```python
from build123d import *

# Parameters (mm, degrees)
BOSS_EXTRUDE1_DEPTH        = 3
BOSS_EXTRUDE1_DEPTH_BACK   = 3
SKETCH2_R                  = 4.5
BOSS_EXTRUDE2_DEPTH        = 8.5
BOSS_EXTRUDE2_DEPTH_BACK   = 8.5
SKETCH2_4_R                = 4.5
BOSS_EXTRUDE3_DEPTH        = 8.5
BOSS_EXTRUDE3_DEPTH_BACK   = 8.5
M3_TAPPED_HOLE1_REACH      = 52.91
M3_TAPPED_HOLE1_BORE_R     = 1.25
M3_TAPPED_HOLE2_REACH      = 52.91
M3_TAPPED_HOLE2_BORE_R     = 1.25
M4_TAPPED_HOLE1_AT_2_COUNT = 2
M4_TAPPED_HOLE1_AT_2_PITCH = 12
M5_TAPPED_HOLE2_AT_2_COUNT = 2
M5_TAPPED_HOLE2_AT_2_PITCH = 12


with BuildPart() as part:
    # Sketch2 → Boss-Extrude1 (new, two sides: drawn at the far end of the back side and taken through both)
    with BuildSketch(Plane(origin=(0, 0, 0), x_dir=(0, 0, -1), z_dir=(1, 0, 0)).offset(-BOSS_EXTRUDE1_DEPTH_BACK)):
        with BuildLine():
            Line((-6, -4.733334115), (20.564415122, -14.401990511))
            ThreePointArc((20.564415122, -14.401990511), (27.686806127, -12.56566856), (28.53576338, -5.259520223))
            ThreePointArc((28.53576338, -5.259520223), (28.211096751, -4.433651902), (28.076506478, -3.556524566))
            ThreePointArc((28.076506478, -3.556524566), (27.692579293, -2.458130667), (26.76223606, -1.759324035))
            Line((26.76223606, -1.759324035), (23.943158198, -0.733263605))
            ThreePointArc((23.943158198, -0.733263605), (23.371504837, -0.615809048), (22.790282203, -0.668376983))
            ThreePointArc((22.790282203, -0.668376983), (21.627836935, -0.773512852), (20.484530213, -0.538603739))
            Line((20.484530213, -0.538603739), (-17.527280829, 13.29656403))
            ThreePointArc((-17.527280829, 13.29656403), (-17.964807448, 14.234842894), (-18.812856048, 14.828652917))
            Line((-18.812856048, 14.828652917), (-21.63193391, 15.854713347))
            ThreePointArc((-21.63193391, 15.854713347), (-22.793802419, 15.917409512), (-23.793941695, 15.322774607))
            ThreePointArc((-23.793941695, 15.322774607), (-24.460850408, 14.737369045), (-25.2404174, 14.313408893))
            ThreePointArc((-25.2404174, 14.313408893), (-29.18584464, 7.14866092), (-23, 1.797461456))
            Line((-23, 1.797461456), (-23, -27.746794345))
            ThreePointArc((-23, -27.746794345), (-21.828427125, -30.57522147), (-19, -31.746794345))
            Line((-19, -31.746794345), (-10, -31.746794345))
            ThreePointArc((-10, -31.746794345), (-7.171572875, -30.57522147), (-6, -27.746794345))
            Line((-6, -27.746794345), (-6, -4.733334115))
        make_face()
        with Locations((22.787546054, -8.293988476)):
            Circle(SKETCH2_R, mode=Mode.SUBTRACT)
        with Locations((-22.787546054, 8.293988476)):
            Circle(SKETCH2_R, mode=Mode.SUBTRACT)
    extrude(amount=BOSS_EXTRUDE1_DEPTH + BOSS_EXTRUDE1_DEPTH_BACK)

    # Sketch2<4> → Boss-Extrude2 (add, two sides: drawn at the far end of the back side and taken through both)
    with BuildSketch(Plane(origin=(0, 0, 0), x_dir=(0, 0, -1), z_dir=(1, 0, 0)).offset(-BOSS_EXTRUDE2_DEPTH_BACK)):
        with BuildLine():
            ThreePointArc((-25.2404174, 14.313408893), (-29.18584464, 7.14866092), (-23, 1.797461456))
            ThreePointArc((-23, 1.797461456), (-17.276544623, 4.847415797), (-17.039328728, 11.328456728))
            ThreePointArc((-17.039328728, 11.328456728), (-17.363995357, 12.15432505), (-17.49858563, 13.031452385))
            ThreePointArc((-17.49858563, 13.031452385), (-17.508509891, 13.164486982), (-17.527280829, 13.29656403))
            ThreePointArc((-17.527280829, 13.29656403), (-17.964807448, 14.234842894), (-18.812856048, 14.828652917))
            Line((-18.812856048, 14.828652917), (-21.63193391, 15.854713347))
            ThreePointArc((-21.63193391, 15.854713347), (-22.793802419, 15.917409512), (-23.793941695, 15.322774607))
            ThreePointArc((-23.793941695, 15.322774607), (-24.460850408, 14.737369045), (-25.2404174, 14.313408893))
        make_face()
        with Locations((-22.787546054, 8.293988476)):
            Circle(SKETCH2_4_R, mode=Mode.SUBTRACT)
    extrude(amount=BOSS_EXTRUDE2_DEPTH + BOSS_EXTRUDE2_DEPTH_BACK)

    # Sketch2<5> → Boss-Extrude3 (add, two sides: drawn at the far end of the back side and taken through both)
    with BuildSketch(Plane(origin=(0, 0, 0), x_dir=(0, 0, -1), z_dir=(1, 0, 0)).offset(-BOSS_EXTRUDE3_DEPTH_BACK)):
        with BuildLine():
            Line((-6, -27.746794345), (-6, -12))
            ThreePointArc((-6, -12), (-7.171572875, -9.171572875), (-10, -8))
            Line((-10, -8), (-19, -8))
            ThreePointArc((-19, -8), (-21.828427125, -9.171572875), (-23, -12))
            Line((-23, -12), (-23, -27.746794345))
            ThreePointArc((-23, -27.746794345), (-21.828427125, -30.57522147), (-19, -31.746794345))
            Line((-19, -31.746794345), (-10, -31.746794345))
            ThreePointArc((-10, -31.746794345), (-7.171572875, -30.57522147), (-6, -27.746794345))
        make_face()
    extrude(amount=BOSS_EXTRUDE3_DEPTH + BOSS_EXTRUDE3_DEPTH_BACK)

    # M3 Tapped Hole1 bore → M3 Tapped Hole1 (cut, up to next)
    with BuildSketch(Plane(origin=(0, 7.047694656, -2.565151075), x_dir=(1, 0, 0), z_dir=(0, 0.9396926207859064, -0.3420201433256741)), mode=Mode.PRIVATE) as m3_tapped_hole1_sk1:
        with Locations((0, -24.25)):
            Circle(M3_TAPPED_HOLE1_BORE_R)
    m3_tapped_hole1_tool1 = extrude(m3_tapped_hole1_sk1.sketch, amount=-M3_TAPPED_HOLE1_REACH, mode=Mode.PRIVATE) & part.part
    add(m3_tapped_hole1_tool1.solids().sort_by_distance((0, 15.341683, 20.222395))[0], mode=Mode.SUBTRACT)

    # M3 Tapped Hole2 bore → M3 Tapped Hole2 (cut, up to next)
    with BuildSketch(Plane(origin=(0, 7.047694656, -2.565151075), x_dir=(1, 0, 0), z_dir=(0, 0.9396926207859064, -0.34202014332567404)), mode=Mode.PRIVATE) as m3_tapped_hole2_sk1:
        with Locations((0, 24.25)):
            Circle(M3_TAPPED_HOLE2_BORE_R)
    m3_tapped_hole2_tool1 = extrude(m3_tapped_hole2_sk1.sketch, amount=-M3_TAPPED_HOLE2_REACH, mode=Mode.PRIVATE) & part.part
    add(m3_tapped_hole2_tool1.solids().sort_by_distance((0, -1.246294, -25.352697))[0], mode=Mode.SUBTRACT)

    # Sketch10 → M4 Tapped Hole1 (revolve, cut)
    with BuildSketch(Plane(origin=(-8.5, -15, 18), x_dir=(0, 0, 1), z_dir=(0, 1, 0))):
        Polygon((0, 0), (0, 17), (1.65, 17), (1.65, 8), (2, 8), (2, 0.025), (2.025, 0), align=None)
    m4_tapped_hole1 = revolve(axis=Axis((-14.85, -15, 18), (1, 0, 0)), mode=Mode.SUBTRACT)

    # M4 Tapped Hole1 at 2: M4 Tapped Hole1 ×2
    with Locations(*[Vector(0, -0.8122328620674102, -0.5833333333333383) * (i * M4_TAPPED_HOLE1_AT_2_PITCH) for i in range(1, M4_TAPPED_HOLE1_AT_2_COUNT)]):
        add(m4_tapped_hole1, mode=Mode.SUBTRACT)

    # Sketch12 → M5 Tapped Hole2 (revolve, cut)
    with BuildSketch(Plane(origin=(8.5, -15, 11), x_dir=(0, 0, -1), z_dir=(0, 1, 0))):
        Polygon((0, 0), (0, 17), (1.65, 17), (1.65, 8), (2, 8), (2, 0.025), (2.025, 0), align=None)
    m5_tapped_hole2 = revolve(axis=Axis((14.85, -15, 11), (-1, 0, 0)), mode=Mode.SUBTRACT)

    # M5 Tapped Hole2 at 2: M5 Tapped Hole2 ×2
    with Locations(*[Vector(0, -0.8122328620674105, 0.5833333333333377) * (i * M5_TAPPED_HOLE2_AT_2_PITCH) for i in range(1, M5_TAPPED_HOLE2_AT_2_COUNT)]):
        add(m5_tapped_hole2, mode=Mode.SUBTRACT)


solid = part.part
```
Here's how the part is built. I have some questions about the finished solid (model axes, mm). A direction names the side the tool comes from. Coordinates: 2 decimals unless noted, no trailing zeros. Write each loop counter-clockwise with the first axis right and the second up, starting at its lowest first coordinate (ties: lowest second). Pieces come first, ordered by that corner, then holes. Notation, with made-up numbers: M 8.25,14.5 L 66.25,14.5 A21 ccw 66.25,31.5 Z; hole C 24,36.25 d8. An arc over 180 degrees is marked long. Answer as CSV lines item,"result". Start each with the question number.
Q1. I need wall thicknesses on probe 1 along Z at (x, y) = (-7, -15); probe 2 along Y at (x, z) = (5.5, 11); probe 3 along Z at (x, y) = (5.5, -15). Which ranges of each line are inside material? Lowest first, please. Write a range as [from, to].
Q2. If we mould it in two halves opening along Y, with no side actions, what happens to faces 1 (the flat face through (0, -9.5, -7.1)), 2 (the flat face through (-1.38, -1.37, -25.69)), 3 (the flat face through (-6, -8, 14))? For each: pulls with the +Y half, pulls with the -Y half, needs draft (parallel to the pull), parting line crosses it, or undercut.
Q3. Suppose I cut it at C-C, the plane z = -11. List the corners of the cut face in (x, y) for me, then the cut area to 3 significant figures.
Q4. Suppose I cut it at A-A, the plane x = -5.5. List the corners of the cut face in (y, z) for me, then the cut area to 3 significant figures.
Q5. Will these pins go through, and if not, where does the flat tip stop? pin 1 Ø1.2 at (y, z) = (-16, 18.5) entering from -X; pin 2 Ø3 at (x, z) = (3.5, 8) entering from -Y; pin 3 Ø14 at (y, z) = (-2, -15.5) entering from -X.
Q6. Suppose I cut it at B-B, the plane z = 11. List the corners of the cut face in (x, y) for me (3 decimals).
Q7. For faces 4 (the cylindrical face through (5.712, -9.203, 7.141)), 5 (the flat face through (0, -16, 23)), 6 (the cylindrical face through (4.543, -25.348, 16.092)), 7 (the flat face through (-2.008, 15.335, 20.203)), which set-ups out of +Z, -Z, +X, -X, +Y, -Y let a thin tool reach every point of the face, with its end or its side?
Entries:
1,probe 1,"z = [6, 9.35], [12.65, 16], [20, 23]"
1,probe 2,"y = [-31.75, -26.4], [-23.1, -17], [-13, -8]"
1,probe 3,"z = [6, 9], [13, 16.35], [19.65, 23]"
2,face 1,"pulls with the -Y half"
2,face 2,"pulls with the +Y half"
2,face 3,"undercut"
3,outline,"M -3,-10.92 L 3,-10.92 L 3,2.91 L -3,2.91 Z"
3,area,"83.0 mm²"
4,outline,"M -31.75,10 A4 ccw -27.75,6 L -12,6 A4 ccw -8,10 L -8,19 A4 ccw -12,23 L -27.75,23 A4 ccw -31.75,19 Z; M 11.33,17.04 A4 cw 13.03,17.5 A2 ccw 14.83,18.81 L 15.85,21.63 A2 ccw 15.32,23.79 A4 cw 14.31,25.24 A6.5 ccw long Z; hole C -24.75,11 d4; hole C -24.75,18 d3.3; hole C -15,18 d4; hole C -15,11 d3.3; hole C 8.29,22.79 d9"
4,area,"425 mm²"
5,pin 1,"stops at x = -0.5"
5,pin 2,"stops at y = -31.72"
5,pin 3,"stops at x = -3"
6,outline,"M -8.5,-31.747 L 8.5,-31.747 L 8.5,-26.397 L -0.5,-26.397 L -0.5,-26.747 L -8.475,-26.747 L -8.5,-26.772 Z; M -8.5,-22.722 L -8.475,-22.747 L -0.5,-22.747 L -0.5,-23.097 L 8.5,-23.097 L 8.5,-17.025 L 8.475,-17 L 0.5,-17 L 0.5,-16.65 L -8.5,-16.65 Z; M -8.5,-13.35 L 0.5,-13.35 L 0.5,-13 L 8.475,-13 L 8.5,-12.975 L 8.5,-8 L 3,-8 L 3,10.921 L -3,10.921 L -3,-8 L -8.5,-8 Z"
7,face 4,"-Z, +X, +Y"
7,face 5,"+Z, +X, -X, -Y"
7,face 6,"+X"
7,face 7,"-Z, +X, -X, +Y"
